Geometry: see drawing. Coordinates: mm, zero at the bounding-box minimum. Give positions to 0.01 mm unless a question says otherwise; leave off trailing zeros. Order: outer loops, then holes, each group sorted by start corner. A loop starts at its lowest first (then second) coordinate and runs counter-clockwise, first axis right, second up. Notation, with made-up numbers: M 4.25,21.5 L 51.25,21.5 A16 ccw 51.25,31.5 Z; hole C 89,82.5 d4. An arc over 180 degrees is marked long. Answer as a JSON object with one key per item and string values. Group by question number.
1. Pin query (flat end, axial travel): P1, Ø4.5, axis at y = 6.5, z = 21.5, coming from the -X side; P2, Ø2, axis at x = 66.5, z = 27.5, coming from the -Y side; P3, Ø4.5, axis at y = 11, z = 23, coming from the +X side; P4, Ø7.5, axis at x = 364, y = 7.5, coming from the -Z side. Return the tip coordinate at first contact, or that it passes through.
2. Section query A-A (z = 24.5). Output: boundary loops of the cut face in (x, y), plus the area to 3 significant figures.
3. Material intervals for L1, parallel to X at y = 6.25, z = 18.5; L2, parallel to X at y = 14, z = 5.5; L3, parallel to X at y = 12.75, z = 24, sorted ascending. Write a range as [from, to].
4. Section query B-B (y = 12.5). Output: boundary loops of the cut face in (x, z).
5. Section query C-C (x = 77.5). Output: boundary loops of the cut face in (y, z), plus the area to 3 significant figures.
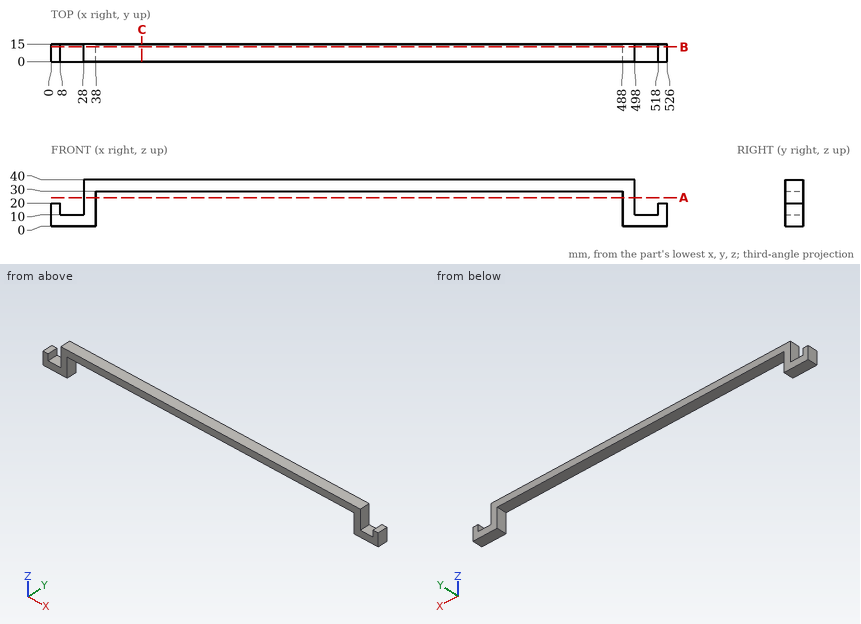
Answer sheet:
{
 "1": {"P1": "x = 0", "P2": "through", "P3": "x = 498", "P4": "z = 30"},
 "2": {"outline": "M 28,0 L 38,0 L 38,15 L 28,15 Z; M 488,0 L 498,0 L 498,15 L 488,15 Z", "area": "300 mm^2"},
 "3": {"L1": "[0, 8], [28, 38], [488, 498], [518, 526]", "L2": "[0, 38], [488, 526]", "L3": "[28, 38], [488, 498]"},
 "4": {"outline": "M 0,0 L 38,0 L 38,30 L 488,30 L 488,0 L 526,0 L 526,20 L 518,20 L 518,10 L 498,10 L 498,40 L 28,40 L 28,10 L 8,10 L 8,20 L 0,20 Z"},
 "5": {"outline": "M 0,30 L 15,30 L 15,40 L 0,40 Z", "area": "150 mm^2"}
}
